The listing builds one solid part. Answer for the finished solid, in the listing's coordinates (mm). A direction names the side the tool comes from. Coordinates: 2 decimals unless noted, no trailing zeros. Order: outer loops, then holes, each group sorted by start corner. A loop starts at its lowest first (then second) coordinate and runs counter-clockwise, first axis right, second up. Notation, with made-up numbers: (-25.75, 72) -> (6.25, 72) arc R8 cw to (6.25, 86) -> close; hole circle Ø7 at (17, -24.75). An arc over 180 degrees is marked (long way). Return JSON: item names as keys, results as strings.
from build123d import *

# Parameters (mm, degrees)
BOSS_EXTRU_1_DEPTH           = 40
ENL_V_MAT_EXTRU_1_DEPTH      = 43.650205158
ENL_V_MAT_EXTRU_1_DEPTH_BACK = 43.650205158
ENL_V_MAT_EXTRU_3_DEPTH      = 40
TROU_TARAUD_M31_D            = 2.5
TROU_TARAUD_M31_DEPTH        = 8.5
TROU_TARAUD_M31_TIP          = 0.751075774
ENL_V_MAT_EXTRU_4_DEPTH      = 3.6


with BuildPart() as part:
    # Esquisse1 → Boss.-Extru.1 (new body)
    with BuildSketch(Plane.XY):
        Polygon((0, -2), (2, 0), (4.8, 0), (4.8, -10.6), (4.43, -11), (5.42, -12.5), (4.43, -14), (1.23, -14), align=None)
    extrude(amount=BOSS_EXTRU_1_DEPTH)

    # Esquisse2 → Enlèv. mat.-Extru.1 (cut, two sides: drawn at the far end of the back side and taken through both)
    with BuildSketch(Plane(origin=(4.8, 0, 0), x_dir=(0, 0, -1), z_dir=(1, 0, 0)).offset(-ENL_V_MAT_EXTRU_1_DEPTH_BACK)):
        Polygon((0, -14), (0, -6.3), (-3, -14), align=None)
    extrude(amount=ENL_V_MAT_EXTRU_1_DEPTH + ENL_V_MAT_EXTRU_1_DEPTH_BACK, mode=Mode.SUBTRACT)

    # Esquisse3 → Enlèv. mat.-Extru.3 (cut)
    with BuildSketch(Plane(origin=(0, -6.5, 0), x_dir=(-1, 0, 0), z_dir=(0, 1, 0))):
        Polygon((-6.8, 40), (-1.3, 40), (-4.8, 36.25), (-6.8, 36.25), align=None)
    extrude(amount=-ENL_V_MAT_EXTRU_3_DEPTH, mode=Mode.SUBTRACT)

    # Trou taraudé M31
    with Locations(Plane(origin=(4.8, 0, 0), x_dir=(0, 0, -1), z_dir=(1, 0, 0))):
        with Locations((-11, -9), (-21, -9)):
            Hole(TROU_TARAUD_M31_D / 2, depth=TROU_TARAUD_M31_DEPTH)
            with Locations((0, 0, -(TROU_TARAUD_M31_DEPTH + TROU_TARAUD_M31_TIP / 2))):  # 118° drill point
                Cone(0, TROU_TARAUD_M31_D / 2, TROU_TARAUD_M31_TIP, mode=Mode.SUBTRACT)

    # Esquisse6 → Enlèv. mat.-Extru.4 (cut)
    with BuildSketch(Plane(origin=(4.8, 0, 0), x_dir=(0, 0, -1), z_dir=(1, 0, 0))):
        with BuildLine():
            Line((-33, -3), (-17, -3))
            ThreePointArc((-17, -3), (-15.5, -4.5), (-17, -6))
            Line((-17, -6), (-33, -6))
            ThreePointArc((-33, -6), (-34.5, -4.5), (-33, -3))
        make_face()
    extrude(amount=-ENL_V_MAT_EXTRU_4_DEPTH, mode=Mode.SUBTRACT)


solid = part.part
1. Determine the mould class of faces 1 (the face through (2.9, -10.1, 1.48)), 2 (the face through (2.652, -7.946, 21.672)), 3 (the face through (4, -6.5, 39)), 4 (the face through (3, -3, 25)) for opening direction Z: pulls with the +Z half, pulls with the -Z half, needs draft (parallel to the pull), parting line crosses it, or undercut.
Answer block:
{"face 1": "pulls with the -Z half", "face 2": "undercut", "face 3": "needs draft", "face 4": "undercut"}
2. For faces 5 (the face through (3, -6, 25)), 6 (the face through (4.8, -6.4, 19.7)), 7 (the face through (4.92, -11.74, 19)), determine the directions among +Z, -Z, +X, -X, +Y, -Y from which every point of the face is accessible in a straight line to the end or side of a thin tool.
Answer block:
{"face 5": "+X", "face 6": "+Z, -Z, +X, +Y", "face 7": "+Z, -Z, +X"}
3. Each of these flat-tipped pins is pushed along its axis until it touches: pin 1 Ø3 at (y, z) = (-9, 21) entering from +X; pin 2 Ø1.5 at (y, z) = (-4, 20.5) entering from +X; pin 3 Ø1 at (y, z) = (-10, 23) entering from -X; pin 4 Ø8 at (y, z) = (-5, 19.5) entering from -X. Where does it stop, or does it pass through?
Answer block:
{"pin 1": "stops at x = 4.8", "pin 2": "stops at x = 1.2", "pin 3": "stops at x = 0.77", "pin 4": "stops at x = 0"}
4. The part is cut by section D-D on y = -4.5. Give the vertices of the cut face in (x, z).
Answer block:
{"outline": "(0.26, 0) -> (4.8, 0) -> (4.8, 15.5) -> (1.2, 15.5) -> (1.2, 34.5) -> (4.8, 34.5) -> (4.8, 40) -> (0.26, 40) -> close"}
5. The part is cut by section C-C on z = 31.5. Give the vertices of the cut face in (x, y), and give its area (3 significant figures).
Answer block:
{"outline": "(0, -2) -> (1.23, -14) -> (4.43, -14) -> (5.42, -12.5) -> (4.43, -11) -> (4.8, -10.6) -> (4.8, -6) -> (1.2, -6) -> (1.2, -3) -> (4.8, -3) -> (4.8, 0) -> (2, 0) -> close", "area": "47.3 mm2"}
6. The part is cut by section A-A on z = 11. Give the vertices of the cut face in (x, y).
Answer block:
{"outline": "(0, -2) -> (0.59, -7.75) -> (4.8, -7.75) -> (4.8, 0) -> (2, 0) -> close; (0.85, -10.25) -> (1.23, -14) -> (4.43, -14) -> (5.42, -12.5) -> (4.43, -11) -> (4.8, -10.6) -> (4.8, -10.25) -> close"}
7. Consider line 1 (Y direction, x = 2.3, z = 21); line 2 (Z direction, x = 3.1, y = -10); line 3 (Z direction, x = 3.2, y = -9). Determine where each line is inside the solid, lowest interval first. Write a range as from..to.
Answer block:
{"line 1": "y = -14..-10.25, -7.75..-6, -3..0", "line 2": "z = 1.44..10.25, 11.75..20.25, 21.75..38.07", "line 3": "z = 1.05..9.75, 12.25..19.75, 22.25..37.96"}
8. The part is cut by section B-B on y = -9. Give the vertices of the cut face in (x, z), and give its area (3 significant figures).
Answer block:
{"outline": "(0.72, 1.05) -> (4.8, 1.05) -> (4.8, 9.75) -> (0.72, 9.75) -> close; (0.72, 12.25) -> (4.8, 12.25) -> (4.8, 19.75) -> (0.72, 19.75) -> close; (0.72, 22.25) -> (4.8, 22.25) -> (4.8, 36.25) -> (1.3, 40) -> (0.72, 40) -> close", "area": "132 mm2"}
